```python
from build123d import *

# Parameters (mm, degrees)
SKETCH1_W           = 50
SKETCH1_H           = 25
BOSS_EXTRUDE1_DEPTH = 25
FILLET2_R           = 5
CUT_EXTRUDE1_DEPTH  = 15
SKETCH3_R           = 2.5
CUT_EXTRUDE2_DEPTH  = 10


with BuildPart() as part:
    # Sketch1 → Boss-Extrude1 (new body)
    with BuildSketch(Plane(origin=(0, 0, 0), x_dir=(1, 0, 0), z_dir=(0, 1, 0))):
        Rectangle(SKETCH1_W, SKETCH1_H)
    extrude(amount=BOSS_EXTRUDE1_DEPTH)

    # Fillet2
    fillet2_edges = [part.edges().sort_by_distance(p)[0] for p in [
        (25, 12.5, 12.5),
        (-25, 12.5, 12.5),
        (-25, 12.5, -12.5),
        (25, 12.5, -12.5),
    ]]
    fillet(fillet2_edges, radius=FILLET2_R)

    # Sketch2 → Cut-Extrude1 (cut)
    with BuildSketch(Plane(origin=(0, 25, 0), x_dir=(1, 0, 0), z_dir=(0, 1, 0))):
        with BuildLine():
            Line((-13.058351702, 9.034247402), (13.06, 9.034247402))
            ThreePointArc((13.06, 9.034247402), (22.094247402, 0), (13.06, -9.034247402))
            Line((13.06, -9.034247402), (-13.058351702, -9.034247402))
            ThreePointArc((-13.058351702, -9.034247402), (-22.092599103, 0), (-13.058351702, 9.034247402))
        make_face()
    extrude(amount=-CUT_EXTRUDE1_DEPTH, mode=Mode.SUBTRACT)

    # Sketch3 → Cut-Extrude2 (cut)
    with BuildSketch(Plane.XY.offset(12.5)):
        with Locations((13.408381173, 13.105781034)):
            Circle(SKETCH3_R)
    extrude(amount=-CUT_EXTRUDE2_DEPTH, mode=Mode.SUBTRACT)


solid = part.part
```
Read the model definition and answer for the solid it produces. Units are mm, in the model's axes. A direction names the side the tool comes from. Coordinates: 2 decimals unless noted, no trailing zeros. Write each loop counter-clockwise with the first axis right and the second up, starting at its lowest first coordinate (ties: lowest second). Pieces come first, ordered by that corner, then holes. Notation, with made-up numbers: (80, -11) -> (139, -11) arc R18 cw to (139, 10) -> close; hole circle Ø11 at (49, 25). An arc over 180 degrees is marked (long way). Answer as a JSON object with one key per item and string values.
Q1. A flat-ended cylindrical pin translates along its axis: pin 1 Ø9 at (x, z) = (-2, -2.5) entering from +Y. Find the tip coordinate at first contact, or state that the pin passes through.
The answers:
{"pin 1": "stops at y = 10"}
Q2. The part is cut by section C-C on z = 0. Give the vertices of the cut face in (x, y).
The answers:
{"outline": "(-25, 0) -> (25, 0) -> (25, 25) -> (22.09, 25) -> (22.09, 10) -> (-22.09, 10) -> (-22.09, 25) -> (-25, 25) -> close"}
Q3. Determine the mould class of faces 1 (the flat face through (25, 12, 0)), 2 (the cylindrical face through (-22.09, 17.6, 0.2)), 3 (the flat face through (0, 10, 0)), 4 (the flat face through (0, 12, 12.5)) for opening direction X: pulls with the +X half, pulls with the -X half, needs draft (parallel to the pull), parting line crosses it, or undercut.
The answers:
{"face 1": "pulls with the +X half", "face 2": "undercut", "face 3": "undercut", "face 4": "needs draft"}
Q4. A tool of negligible diameter and unlimited length cuts with its end or side. For faces 5 (the flat face through (0, 0, 0)), 6 (the flat face through (0, 18, 9.034)), 7 (the cylindrical face through (15.79, 13.86, 10.56)), from which of +Z, -Z, +X, -X, +Y, -Y can it reach the whole face along a straight path? Write none if from no direction.
The answers:
{"face 5": "+Z, -Z, +X, -X, -Y", "face 6": "+Y", "face 7": "+Z"}
Q5. The part is cut by section B-B on x = 12. Give the vertices of the cut face in (y, z), then the cut area to 3 significant figures.
The answers:
{"outline": "(0, -12.5) -> (25, -12.5) -> (25, -9.03) -> (10, -9.03) -> (10, 9.03) -> (11.04, 9.03) -> (11.04, 12.5) -> (0, 12.5) -> close; (15.17, 9.03) -> (25, 9.03) -> (25, 12.5) -> (15.17, 12.5) -> close", "area": "340 mm2"}
Q6. The part is cut by section A-A on y = 23.25. Give the vertices of the cut face in (x, z).
The answers:
{"outline": "(-25, -7.5) arc R5 ccw to (-20, -12.5) -> (20, -12.5) arc R5 ccw to (25, -7.5) -> (25, 7.5) arc R5 ccw to (20, 12.5) -> (-20, 12.5) arc R5 ccw to (-25, 7.5) -> close; hole (-13.06, -9.03) -> (13.06, -9.03) arc R9.03 ccw to (13.06, 9.03) -> (-13.06, 9.03) arc R9.03 ccw to start"}
Q7. Consider line 1 (Y direction, x = 14.5, z = 6); line 2 (Z direction, x = 2, y = 16.25); line 3 (X direction, y = 14.25, z = 6.5). Determine where each line is inside the solid, lowest interval first. Write a range as [from, to].
The answers:
{"line 1": "y = [0, 10]", "line 2": "z = [-12.5, -9.03], [9.03, 12.5]", "line 3": "x = [-25, -19.33], [19.33, 25]"}
Q8. The part is cut by section D-D on y = 3. Give the vertices of the cut face in (x, z).
The answers:
{"outline": "(-25, -7.5) arc R5 ccw to (-20, -12.5) -> (20, -12.5) arc R5 ccw to (25, -7.5) -> (25, 7.5) arc R5 ccw to (20, 12.5) -> (-20, 12.5) arc R5 ccw to (-25, 7.5) -> close"}
